Source: CAD feature listing. Evaluate the final solid. Frame: model axes, mm. A direction names the side the tool comes from. Give positions to 0.01 mm unless a question says otherwise; leave off trailing zeros. Loops run counter-clockwise (first coordinate to the right, second up) from the corner with the lowest first, then second, coordinate; pieces in that order, holes last. Notation, with made-up numbers: M -1,15 L 8,15 A21 cw 8,54 Z; hole C -28,47.5 d9. An arc over 180 degrees is marked long. Put each result on its own line as item: value.
from build123d import *

# Parameters (mm, degrees)
PAD006_DEPTH    = 18
SKETCH017_W     = 17.45
SKETCH017_H     = 2.4
POCKET010_DEPTH = 6.75
SKETCH018_W     = 5.63
SKETCH018_H     = 7.8
PAD007_DEPTH    = 0.66


with BuildPart() as part:
    # Sketch016 → Pad006 (new body)
    with BuildSketch(Plane.XZ):
        Polygon((21.151384, 8.480667), (15.151384, 9.360667), (15.151384, 8.760667), (6.701384, 10), (6.701384, 5.25), (5.201384, 5.25), (5.201384, 4.25), (11.74, 4.25), (11.74, 3.5), (17.37, 3.5), (17.37, 4.25), (22.651384, 4.25), (22.651384, 5.25), (21.151384, 5.25), align=None)
    extrude(amount=PAD006_DEPTH)

    # Sketch017 → Pocket010 (cut)
    with BuildSketch(Plane.XY.offset(12)):
        with Locations((13.926384, -9)):
            Rectangle(SKETCH017_W, SKETCH017_H)
    extrude(amount=-POCKET010_DEPTH, mode=Mode.SUBTRACT)

    # Sketch018 (on Face13 of Pocket010) → Pad007 (join)
    with BuildSketch(Plane(origin=(0, 0, 3.5), x_dir=(1, 0, 0), z_dir=(0, 0, -1))):
        with Locations((14.555, 14.1)):
            Rectangle(SKETCH018_W, SKETCH018_H)
    extrude(amount=PAD007_DEPTH)


with BuildPart() as part_1:
    # Body003 placement: moved
    add(part.part.moved(Location((0, -37.5, 0))))


solid = part_1.part
1. Draft query along X for faces 1 (the flat face through (11.74, -48, 4)), 2 (the flat face through (14, -45.3, 7)), 3 (the flat face through (10.99, -41.35, 9.37)). Return one class per face: pulls with the +X half, pulls with the -X half, needs draft (parallel to the pull), parting line crosses it, or undercut.
Found:
face 1: pulls with the -X half
face 2: needs draft
face 3: undercut
2. Access query for faces 4 (the flat face through (17.37, -48, 4)), 5 (the flat face through (8, -46, 4.25)), 6 (the flat face through (21.151, -52, 7)), 7 (the flat face through (6.701, -52, 8)). Directions: +Z, -Z, +X, -X, +Y, -Y. A direction counts if a zero-diameter tool reaches every point of the face in a straight line with its end or side. Return the directions, or none.
Found:
face 4: -Z, +X, +Y, -Y
face 5: -Z, -X, +Y, -Y
face 6: +Z, +X, +Y, -Y
face 7: +Z, -X, +Y, -Y
3. Section query B-B (y = -45). Output: boundary loops of the cut face in (x, z), plus the area to 3 significant figures.
Found:
outline: M 5.2,4.25 L 11.74,4.25 L 11.74,3.5 L 17.37,3.5 L 17.37,4.25 L 22.65,4.25 L 22.65,5.25 L 21.15,5.25 L 21.15,8.48 L 15.15,9.36 L 15.15,8.76 L 6.7,10 L 6.7,5.25 L 5.2,5.25 Z
area: 78.6 mm^2
4. Section query A-A (z = 7.75). Output: boundary loops of the cut face in (x, y), plus the area to 3 significant figures.
Found:
outline: M 6.7,-55.5 L 21.15,-55.5 L 21.15,-47.7 L 6.7,-47.7 Z; M 6.7,-45.3 L 21.15,-45.3 L 21.15,-37.5 L 6.7,-37.5 Z
area: 225 mm^2
5. Material intervals for line 1 (Y direction, x = 19.25, z = 5.75); line 2 (X direction, y = -49, z = 3.75); line 3 (Z direction, x = 15.5, y = -47.5), sorted ascending. Write a range as from..to.
Found:
line 1: -55.5..-47.7, -45.3..-37.5
line 2: 11.74..17.37
line 3: 3.5..5.25
6. Section query C-C (x = 19). Output: boundary loops of the cut face in (y, z).
Found:
outline: M -55.5,4.25 L -37.5,4.25 L -37.5,8.8 L -45.3,8.8 L -45.3,5.25 L -47.7,5.25 L -47.7,8.8 L -55.5,8.8 Z
7. Section query D-D (y = -47.25). Output: boundary loops of the cut face in (x, z), plus the area to 3 significant figures.
Found:
outline: M 5.2,4.25 L 11.74,4.25 L 11.74,3.5 L 17.37,3.5 L 17.37,4.25 L 22.65,4.25 L 22.65,5.25 L 5.2,5.25 Z
area: 21.7 mm^2
8. Contact query for flat-ended pins moving along their axis: P1, Ø5, axis at x = 9, y = -50.5, coming from the -Z side; P2, Ø2.5, axis at y = -50.5, z = 7, coming from the -X side; P3, Ø8.5, axis at x = 11, y = -50, coming from the +Z side; P4, Ø8, axis at x = 20, y = -50, coming from the -Z side. Output: stop coordinate, or through.
Found:
P1: z = 4.25
P2: x = 6.7
P3: z = 9.99
P4: z = 2.84
